```python
from build123d import *

# Parameters (mm, degrees)
F0_W     = 1066.8
F0_H     = 342.9
F1_DEPTH = 50.8
F2_W     = 41.275
F2_H     = 60.325
F3_DEPTH = 50.8
F4_R     = 38.1


with BuildPart() as f1:
    # F0 (on Top) → F1 (new body)
    with BuildSketch(Plane.XY):
        Rectangle(F0_W, F0_H)
    extrude(amount=F1_DEPTH)

    # F2 (on face) → F3 (cut)
    with BuildSketch(Plane.XY.offset(50.8)):
        Polygon((-317.5, -114.3), (-317.5, -171.45), (-285.75, -171.45), (-285.75, -101.6), (-327.025, -101.6), (-327.025, 139.7), (-365.125, 139.7), (-403.225, 101.537321), (-403.225, 31.75), (-501.65, 31.75), (-501.65, 0), (-403.225, 0), (-403.225, -114.3), align=None)
        with Locations((-49.2125, 14.2875)):
            Rectangle(F2_W, F2_H)
    extrude(amount=-F3_DEPTH, mode=Mode.SUBTRACT)

    # F4
    f4_edges = [f1.edges().sort_by_distance(p)[0] for p in [
        (-533.4, 171.45, 25.4),
        (-533.4, -171.45, 25.4),
        (533.4, 171.45, 25.4),
        (533.4, -171.45, 25.4),
    ]]
    fillet(f4_edges, radius=F4_R)


solid = f1.part
```
Part model, mm, in its own coordinate system. A direction names the side the tool comes from. Round coordinates to 2 decimals unless told otherwise and drop trailing zeros. Write each loop counter-clockwise with the first axis right and the second up, starting at its lowest first coordinate (ties: lowest second). Pieces come first, ordered by that corner, then holes. Notation, with made-up numbers: M 56.5,66 L 83.5,66 A16 ccw 83.5,91 Z; hole C 4,60.5 d11. An arc over 180 degrees is marked long. Answer as CSV lines item,"result". Start each with the question number.
1) Band-saw the part on C-C (z = 8). List the corners of the cut face in (x, y) (3 decimals).
2) Band-saw the part on A-A (y = -92). List the corners of the cut face in (x, z) (3 decimals), then the cut area to 3 significant figures.
3) Mould opens along X. For faces 4 (the face through (522.54, -159.99, 25.76)), 5 (the face through (-383.908, 120.886, 25.756)), 6 (the face through (-522.54, -159.99, 25.76)), 7 (the face through (-453, 0, 26)) say: +X half, -X half, draft (parallel to the pull), parting line (faces both ways), or undercut.
4) Band-saw the part on B-B (x = -439). List the corners of the cut face in (y, z).
5) Drill centre lines: L1, parallel to X at y = 35.5, z = 27 (3 decimals); L2, parallel to X at y = -39, z = 17.5 (3 decimals); L3, parallel to X at y = -127, z = 10. Where is each one in solid material? Low to high.
6) Drop a flat-ended pin along its axis: pin 1 (8 mm diameter, centred on x = -195.5, y = 82.5, fed in from -Z). Give the stop position or say it passes through.
7) Which spindle directions (+Z, -Z, +X, -X, +Y, -Y) get a long thin tool onto all of the face, cutting with end or side? Do faces 1 (the face through (-285.75, -137, 26)), 2 (the face through (-306, -101.6, 26)), 3 (the face through (533.4, -2, 25)). Say none if no direction does.
Worked out:
1,outline,"M -533.4,-133.35 A38.1 ccw -495.3,-171.45 L -317.5,-171.45 L -317.5,-114.3 L -403.225,-114.3 L -403.225,0 L -501.65,0 L -501.65,31.75 L -403.225,31.75 L -403.225,101.537 L -365.125,139.7 L -327.025,139.7 L -327.025,-101.6 L -285.75,-101.6 L -285.75,-171.45 L 495.3,-171.45 A38.1 ccw 533.4,-133.35 L 533.4,133.35 A38.1 ccw 495.3,171.45 L -495.3,171.45 A38.1 ccw -533.4,133.35 Z; hole M -69.85,-15.875 L -28.575,-15.875 L -28.575,44.45 L -69.85,44.45 Z"
2,outline,"M -533.4,0 L -403.225,0 L -403.225,50.8 L -533.4,50.8 Z; M -327.025,0 L 533.4,0 L 533.4,50.8 L -327.025,50.8 Z"
2,area,"50,300 mm²"
3,face 4,"+X half"
3,face 5,"undercut"
3,face 6,"-X half"
3,face 7,"undercut"
4,outline,"M -171.45,0 L 0,0 L 0,50.8 L -171.45,50.8 Z; M 31.75,0 L 171.45,0 L 171.45,50.8 L 31.75,50.8 Z"
5,L1,"-533.4 to -403.225, -327.025 to -69.85, -28.575 to 533.4"
5,L2,"-533.4 to -403.225, -327.025 to 533.4"
5,L3,"-533.4 to -317.5, -285.75 to 533.4"
6,pin 1,"z = 0"
7,face 1,"+Z, -Z, -Y"
7,face 2,"+Z, -Z"
7,face 3,"+Z, -Z, +X, +Y, -Y"
